from build123d import *

# Parameters (mm, degrees)
BASE_SHAPE_DEPTH           = 12
FILLETS_R                  = 1
INSIDE_CUT_DEPTH           = 11
SKETCH3_R                  = 1.625
SKETCH3_R_2                = 3.125
MOUNTING_POSTS_DEPTH       = 10
CENTER_REINFORCEMENT_DEPTH = 1
REINFORCEMENT_FILLETS_R    = 3


with BuildPart() as part:
    # Sketch1 → Base shape (new body)
    with BuildSketch(Plane(origin=(0, 0, 0), x_dir=(1, 0, 0), z_dir=(0, 1, 0))):
        with BuildLine():
            ThreePointArc((2.7, 36.88), (1.909188309, 34.970811691), (0, 34.18))
            Line((0, 34.18), (-73.452025159, 34.18))
            Line((-73.452025159, 34.18), (-73.452025159, 24.62))
            ThreePointArc((-73.452025159, 24.62), (-71.54283685, 23.829188309), (-70.752025159, 21.92))
            ThreePointArc((-70.752025159, 21.92), (-71.54283685, 20.010811691), (-73.452025159, 19.22))
            Line((-73.452025159, 19.22), (-73.452025159, 15.845601913))
            ThreePointArc((-73.452025159, 15.845601913), (-64.231671709, 10.194263093), (-60.622025159, 0))
            ThreePointArc((-60.622025159, 0), (-64.231671709, -10.194263093), (-73.452025159, -15.845601913))
            Line((-73.452025159, -15.845601913), (-73.452025159, -19.22))
            ThreePointArc((-73.452025159, -19.22), (-71.54283685, -20.010811691), (-70.752025159, -21.92))
            ThreePointArc((-70.752025159, -21.92), (-71.54283685, -23.829188309), (-73.452025159, -24.62))
            Line((-73.452025159, -24.62), (-73.452025159, -34.18))
            Line((-73.452025159, -34.18), (0, -34.18))
            ThreePointArc((0, -34.18), (1.909188309, -34.970811691), (2.7, -36.88))
            ThreePointArc((2.7, -36.88), (2.127372404, -38.542614403), (0.652380257, -39.5))
            Line((0.652380257, -39.5), (11.4, -39.5))
            Line((11.4, -39.5), (11.4, 39.5))
            Line((11.4, 39.5), (0.652380257, 39.5))
            ThreePointArc((0.652380257, 39.5), (2.127372404, 38.542614403), (2.7, 36.88))
        make_face()
    extrude(amount=BASE_SHAPE_DEPTH)

    # Fillets
    fillets_edges = [part.edges().sort_by_distance(p)[0] for p in [
        (0.652380257, 6, -39.5),
        (0.652380257, 6, 39.5),
    ]]
    fillet(fillets_edges, radius=FILLETS_R)

    # Sketch2 → Inside cut (cut)
    with BuildSketch(Plane(origin=(0, 12, 0), x_dir=(1, 0, 0), z_dir=(0, 1, 0))):
        with BuildLine():
            Line((10.4, 38.5), (3.326499662, 38.5))
            ThreePointArc((3.326499662, 38.5), (3.1371962, 34.918368026), (0, 33.18))
            Line((0, 33.18), (-72.452025159, 33.18))
            Line((-72.452025159, 33.18), (-72.452025159, 25.482302626))
            ThreePointArc((-72.452025159, 25.482302626), (-69.752025159, 21.92), (-72.452025159, 18.357697374))
            Line((-72.452025159, 18.357697374), (-72.452025159, 16.635597374))
            ThreePointArc((-72.452025159, 16.635597374), (-59.622025159, 0), (-72.452025159, -16.635597374))
            Line((-72.452025159, -16.635597374), (-72.452025159, -18.357697374))
            ThreePointArc((-72.452025159, -18.357697374), (-69.752025159, -21.92), (-72.452025159, -25.482302626))
            Line((-72.452025159, -25.482302626), (-72.452025159, -33.18))
            Line((-72.452025159, -33.18), (0, -33.18))
            ThreePointArc((0, -33.18), (3.1371962, -34.918368026), (3.326499662, -38.5))
            Line((3.326499662, -38.5), (10.4, -38.5))
            Line((10.4, -38.5), (10.4, 38.5))
        make_face()
    extrude(amount=-INSIDE_CUT_DEPTH, mode=Mode.SUBTRACT)

    # Sketch3 → Mounting posts (add)
    with BuildSketch(Plane(origin=(0, 1, 0), x_dir=(1, 0, 0), z_dir=(0, 1, 0))):
        with BuildLine():
            Line((-72.452025159, 26.18), (-68.952025159, 26.18))
            ThreePointArc((-68.952025159, 26.18), (-66.477151425, 27.205126266), (-65.452025159, 29.68))
            Line((-65.452025159, 29.68), (-65.452025159, 33.18))
            Line((-65.452025159, 33.18), (-72.452025159, 33.18))
            Line((-72.452025159, 33.18), (-72.452025159, 26.18))
        make_face()
        with Locations((-68.952025159, 29.68)):
            Circle(SKETCH3_R, mode=Mode.SUBTRACT)
        with BuildLine():
            ThreePointArc((3.384479038, 35.38490748), (4.255839604, 32.665174116), (6.863249831, 31.5))
            Line((6.863249831, 31.5), (10.4, 31.5))
            Line((10.4, 31.5), (10.4, 38.5))
            Line((10.4, 38.5), (3.326499662, 38.5))
            ThreePointArc((3.326499662, 38.5), (3.699359286, 36.948853988), (3.384479038, 35.38490748))
        make_face()
        with Locations((6.863249831, 35)):
            Circle(SKETCH3_R, mode=Mode.SUBTRACT)
        with BuildLine():
            Line((-56.497025159, 3.125), (-59.908291834, 3.125))
            ThreePointArc((-59.908291834, 3.125), (-59.622025159, 0), (-59.908291834, -3.125))
            Line((-59.908291834, -3.125), (-56.497025159, -3.125))
            ThreePointArc((-56.497025159, -3.125), (-53.372025159, 0), (-56.497025159, 3.125))
        make_face()
        with Locations((-56.497025159, 0)):
            Circle(SKETCH3_R, mode=Mode.SUBTRACT)
        with BuildLine():
            Line((10.4, -38.5), (10.4, -31.5))
            Line((10.4, -31.5), (6.863249831, -31.5))
            ThreePointArc((6.863249831, -31.5), (4.255839604, -32.665174116), (3.384479038, -35.38490748))
            ThreePointArc((3.384479038, -35.38490748), (3.699359286, -36.948853988), (3.326499662, -38.5))
            Line((3.326499662, -38.5), (10.4, -38.5))
        make_face()
        with Locations((6.863249831, -35)):
            Circle(SKETCH3_R, mode=Mode.SUBTRACT)
        with BuildLine():
            Line((-68.952025159, -26.18), (-72.452025159, -26.18))
            Line((-72.452025159, -26.18), (-72.452025159, -33.18))
            Line((-72.452025159, -33.18), (-65.452025159, -33.18))
            Line((-65.452025159, -33.18), (-65.452025159, -29.68))
            ThreePointArc((-65.452025159, -29.68), (-66.477151425, -27.205126266), (-68.952025159, -26.18))
        make_face()
        with Locations((-68.952025159, -29.68)):
            Circle(SKETCH3_R, mode=Mode.SUBTRACT)
        with Locations((-24.61101258, 0)):
            Circle(SKETCH3_R_2)
        with Locations((-24.61101258, 0)):
            Circle(SKETCH3_R, mode=Mode.SUBTRACT)
    extrude(amount=MOUNTING_POSTS_DEPTH)

    # Sketch4 → Center reinforcement (add)
    with BuildSketch(Plane(origin=(0, 1, 0), x_dir=(1, 0, 0), z_dir=(0, 1, 0))):
        with BuildLine():
            Line((-27.012184169, 2), (-54.09585357, 2))
            ThreePointArc((-54.09585357, 2), (-53.372025159, 0), (-54.09585357, -2))
            Line((-54.09585357, -2), (-27.012184169, -2))
            ThreePointArc((-27.012184169, -2), (-27.73601258, 0), (-27.012184169, 2))
        make_face()
        with BuildLine():
            Line((10.4, 2), (-22.209840991, 2))
            ThreePointArc((-22.209840991, 2), (-21.672536255, 1.063476324), (-21.48601258, 0))
            ThreePointArc((-21.48601258, 0), (-21.672536255, -1.063476324), (-22.209840991, -2))
            Line((-22.209840991, -2), (10.4, -2))
            Line((10.4, -2), (10.4, 2))
        make_face()
    extrude(amount=CENTER_REINFORCEMENT_DEPTH)

    # Reinforcement fillets
    reinforcement_fillets_edges = [part.edges().sort_by_distance(p)[0] for p in [
        (-53.372025159, 2, 0),
        (-27.73601258, 2, 0),
        (-21.672536255, 2, 1.063476324),
        (10.4, 2, 0),
    ]]
    fillet(reinforcement_fillets_edges, radius=REINFORCEMENT_FILLETS_R)


solid = part.part
The model under review builds one solid part; all positions refer to its coordinate system, in mm. A direction names the side the tool comes from. Round coordinates to 2 decimals unless told otherwise and drop trailing zeros. Loops run counter-clockwise (first coordinate to the right, second up) from the corner with the lowest first, then second, coordinate; pieces in that order, holes last. Notation, with made-up numbers: (79, -23) -> (126, -23) arc R22 ccw to (126, -3) -> close; hole circle Ø9 at (12, 10). An arc over 180 degrees is marked (long way). Return JSON: item names as keys, results as strings.
(1) For pin 1 (1.6 mm diameter, centred on x = 7, z = 35.5, fed in from +Y); pin 2 (5 mm diameter, centred on y = 3.5, z = -10, fed in from -X); pin 3 (1 mm diameter, centred on x = -71, y = 7.5, fed in from +Z), all flat-tipped, find the tip position at first contact; note any pin that passes through.
Solved:
{"pin 1": "y = 1", "pin 2": "x = -66.52", "pin 3": "z = 34.18"}
(2) The part is to be moulded in two halves that separate along X. For faces 4 (the flat face through (-73.452, 6, -18)), 5 (the flat face through (7, 1, -35)), 6 (the flat face through (-32, 0, -1)), say which applies: released by +X, released by -X, zero draft, split by the parting line, or undercut.
Solved:
{"face 4": "released by -X", "face 5": "undercut", "face 6": "zero draft"}
(3) Add section C-C on y = 7. State how many separate pieces and enclosed holes the cut face has, plus the area to 3 significant figures.
Solved:
{"separate pieces": "2", "enclosed holes": "7", "area": "540 mm2"}
(4) Add section B-B on z = -10. Write out the cut boundary in (x, y).
Solved:
{"outline": "(-64.08, 0) -> (11.4, 0) -> (11.4, 12) -> (10.4, 12) -> (10.4, 1) -> (-62.83, 1) -> (-62.83, 12) -> (-64.08, 12) -> close"}
(5) Add section A-A on x = -8.5. Write out the cut boundary in (y, z), plus the area to 3 significant figures.
Solved:
{"outline": "(0, -34.18) -> (12, -34.18) -> (12, -33.18) -> (1, -33.18) -> (1, -2) -> (2, -2) -> (2, 2) -> (1, 2) -> (1, 33.18) -> (12, 33.18) -> (12, 34.18) -> (0, 34.18) -> close", "area": "94.4 mm2"}
(6) For line 1 (X direction, y = 6.75, z = 29.68); line 2 (Z direction, x = -38, y = 6); line 3 (Z direction, x = -55.5, y = 8.25), list the stretches that pass through material, from the lowest coordinate up.
Solved:
{"line 1": "-73.45 to -70.58, -67.33 to -65.45, 10.4 to 11.4", "line 2": "-34.18 to -33.18, 33.18 to 34.18", "line 3": "-34.18 to -33.18, -2.96 to -1.28, 1.28 to 2.96, 33.18 to 34.18"}
(7) For faces 1 (the flat face through (-37, 6, 34.18)), 2 (the flat face through (-73.452, 6, 29)), 3 (the flat face through (-65.452, 6, 31)), list the 3-axis set-ups (+Z, -Z, +X, -X, +Y, -Y) from which the entire face can be reached by the end or side of a thin tool; tool diameter is ignored.
Solved:
{"face 1": "+Z, -X, +Y, -Y", "face 2": "+Z, -Z, -X, +Y, -Y", "face 3": "+Y"}
